Read the model definition and answer for the solid it produces. Units are mm, in the model's axes. A direction names the side the tool comes from. Coordinates: 2 decimals unless noted, no trailing zeros. Loops run counter-clockwise (first coordinate to the right, second up) from the corner with the lowest first, then second, coordinate; pieces in that order, holes last. Notation, with made-up numbers: M 78,53 L 111,53 A22 ccw 111,68 Z; hole C 5.5,35 d7. An arc over 180 degrees is marked long. One line per item, written item: value. Start each with the question number.
1. The part is cut by section C-C (x = 8). Write down the section's boundary in (y, z).
2. The part is cut by section A-A (z = 68). Write down the section's boundary in (x, y), then the cut area to 3 significant figures.
3. The part is cut by section D-D (y = 99.5). State how many separate pieces and enclosed holes the cut face has, then the cut area to 3 significant figures.
4. Flat-ended cylindrical pins translate along their axes: pin 1 (5 mm diameter, centred on y = 79, z = 107.5, fed in from +X); pin 2 (11 mm diameter, centred on y = 51, z = 4, fed in from -X); pin 3 (3 mm diameter, centred on x = -66, z = 4.5, fed in from -Y). Find the tip coordinate at first contact, or state that the pin passes through.
5. The part is cut by section B-B (y = 38.5). Write down the section's boundary in (x, z).
6. For faces 1 (the face through (105.5, 123, 56)), 2 (the face through (-107.31, 117.64, 54.37)), 3 (the face through (34.82, 9.8, 54.7)), 4 (the face through (-64.32, 94.74, 4.93)), determine the directions among +Z, -Z, +X, -X, +Y, -Y from which every point of the face is accessible in a straight line to the end or side of a thin tool.
7. Determine the mould class of faces 5 (the face through (67.53, 95.51, 4.93)), 6 (the face through (34.82, 95, 5)), 7 (the face through (32, 0, 54)), 8 (the face through (-115.5, 125, 54)) for opening direction Y: +Y half, -Y half, draft (parallel to the pull), parting line (faces both ways), or undercut.
8. Consider probe 1 along Z at (x, y) = (27.5, 19); probe 2 along X at (y, z) = (114, 38); probe 3 along Y at (x, z) = (73, 103). Determine where each line is inside the solid, lowest interval first.
```python
from build123d import *

# Parameters (mm, degrees)
SKETCH3_W           = 45.820005247
SKETCH3_H           = 110
EXTRUDE1_DEPTH      = 110
SKETCH5_W           = 90
SKETCH5_H           = 37.77
CUT_EXTRUDE1_DEPTH  = 72
SKETCH6_W           = 45.820005247
SKETCH6_H           = 90
CUT_EXTRUDE3_DEPTH  = 130
SKETCH8_W           = 211
SKETCH8_H           = 90
CUT_EXTRUDE4_DEPTH  = 20
SKETCH9_W           = 91.800610731
SKETCH9_H           = 90
CUT_EXTRUDE6_DEPTH  = 10
SKETCH10_W          = 90
SKETCH10_H          = 72.23
CUT_EXTRUDE9_DEPTH  = 10
SKETCH11_W          = 103.619303527
SKETCH11_H          = 90
CUT_EXTRUDE11_DEPTH = 20
SKETCH12_W          = 90
SKETCH12_H          = 82.03288143
CUT_EXTRUDE13_DEPTH = 20


with BuildPart() as part:
    # Sketch3 → Extrude1 (new body)
    with BuildSketch(Plane.XY):
        Polygon((-115.5, 130), (115.5, 130), (115.5, 120), (34.820005247, 57.918579334), (34.820005247, 0), (-31, 0), (-31, 57.77), (-115.5, 120), align=None)
        Polygon((-31, 120), (-31, 70.171133991), (-98.581267218, 120), align=None, mode=Mode.SUBTRACT)
        Polygon((34.820005247, 70.319713325), (34.820005247, 120), (99.331172327, 120), align=None, mode=Mode.SUBTRACT)
        with Locations((1.910002624, 65)):
            Rectangle(SKETCH3_W, SKETCH3_H, mode=Mode.SUBTRACT)
    extrude(amount=EXTRUDE1_DEPTH)

    # Sketch5 → Cut-Extrude1 (cut)
    with BuildSketch(Plane.ZY.offset(31)):
        with Locations((55, 28.885)):
            Rectangle(SKETCH5_W, SKETCH5_H)
    extrude(amount=-CUT_EXTRUDE1_DEPTH, mode=Mode.SUBTRACT)

    # Sketch6 → Cut-Extrude3 (cut)
    with BuildSketch(Plane(origin=(0, 0, 0), x_dir=(1, 0, 0), z_dir=(0, 1, 0))):
        with Locations((1.910002624, -55)):
            Rectangle(SKETCH6_W, SKETCH6_H)
    extrude(amount=CUT_EXTRUDE3_DEPTH, mode=Mode.SUBTRACT)

    # Sketch8 → Cut-Extrude4 (cut)
    with BuildSketch(Plane(origin=(0, 130, 0), x_dir=(1, 0, 0), z_dir=(0, 1, 0))):
        with Locations((0, -55)):
            Rectangle(SKETCH8_W, SKETCH8_H)
    extrude(amount=-CUT_EXTRUDE4_DEPTH, mode=Mode.SUBTRACT)

    # Sketch9 → Cut-Extrude6 (cut)
    with BuildSketch(Plane(origin=(-15.043239393, 19.549946865, 0), x_dir=(0.792529575, 0.60983348, 0), z_dir=(0.60983348, -0.792529575, 0))):
        with Locations((108.816878092, 55)):
            Rectangle(SKETCH9_W, SKETCH9_H)
    extrude(amount=-CUT_EXTRUDE6_DEPTH, mode=Mode.SUBTRACT)

    # Sketch10 → Cut-Extrude9 (cut)
    with BuildSketch(Plane(origin=(34.820005247, 0, 0), x_dir=(0, 0, -1), z_dir=(1, 0, 0))):
        with Locations((-55, 83.885)):
            Rectangle(SKETCH10_W, SKETCH10_H)
    extrude(amount=-CUT_EXTRUDE9_DEPTH, mode=Mode.SUBTRACT)

    # Sketch11 → Cut-Extrude11 (cut)
    with BuildSketch(Plane(origin=(16.683281999, 22.653661079, 0), x_dir=(0.805206703, -0.592994238, 0), z_dir=(-0.592994238, -0.805206703, 0))):
        with Locations((-104.356929468, 55)):
            Rectangle(SKETCH11_W, SKETCH11_H)
    extrude(amount=-CUT_EXTRUDE11_DEPTH, mode=Mode.SUBTRACT)

    # Sketch12 → Cut-Extrude13 (cut)
    with BuildSketch(Plane.ZY.offset(31)):
        with Locations((55, 88.786440715)):
            Rectangle(SKETCH12_W, SKETCH12_H)
    extrude(amount=-CUT_EXTRUDE13_DEPTH, mode=Mode.SUBTRACT)


solid = part.part
```
Answer block:
1. outline: M 0,0 L 10,0 L 10,10 L 0,10 Z; M 0,100 L 10,100 L 10,110 L 0,110 Z; M 120,0 L 130,0 L 130,10 L 120,10 Z; M 120,100 L 130,100 L 130,110 L 120,110 Z
2. outline: M -115.5,120 L -109.06,115.26 L -105.5,120.1 L -105.5,130 L -115.5,130 Z; M -31,0 L -21,0 L -21,10 L -31,10 Z; M 24.82,0 L 34.82,0 L 34.82,10 L 24.82,10 Z; M 105.5,116.6 L 107.57,113.9 L 115.5,120 L 115.5,130 L 105.5,130 Z
2. area: 458 mm2
3. separate pieces: 8
3. enclosed holes: 0
3. area: 1,060 mm2
4. pin 1: stops at x = 65.47
4. pin 2: stops at x = -31
4. pin 3: stops at y = 82.44
5. outline: M -31,0 L -21,0 L -21,10 L -31,10 Z; M -31,100 L -21,100 L -21,110 L -31,110 Z; M 24.82,0 L 34.82,0 L 34.82,10 L 24.82,10 Z; M 24.82,100 L 34.82,100 L 34.82,110 L 24.82,110 Z
6. face 1: +Y, -Y
6. face 2: -Y
6. face 3: +Z, -Z, +X, -Y
6. face 4: +Z, -Z
7. face 5: undercut
7. face 6: undercut
7. face 7: -Y half
7. face 8: draft
8. probe 1: z = 0 to 10, 100 to 110
8. probe 2: x = 107.5 to 107.7
8. probe 3: y = 87.3 to 99.72, 120 to 130
